Work out the finished part from the listing and answer in its coordinate system (mm). Face numbers are marked on the shaded views. A direction names the side the tool comes from. Give positions to 0.01 mm unless a question says otherwise; leave off trailing zeros. Loops run counter-clockwise (first coordinate to the right, second up) from the corner with the lowest first, then second, coordinate; pieces in that order, holes last. Notation, with made-up numbers: (84.5, -20.75) - (129.5, -20.75) arc R22 ccw to (129.5, 16.25) - close; hole circle Ø3 at (-26, 29). An arc over 180 degrees is marked (long way). One line per question, with ' | ' between items.
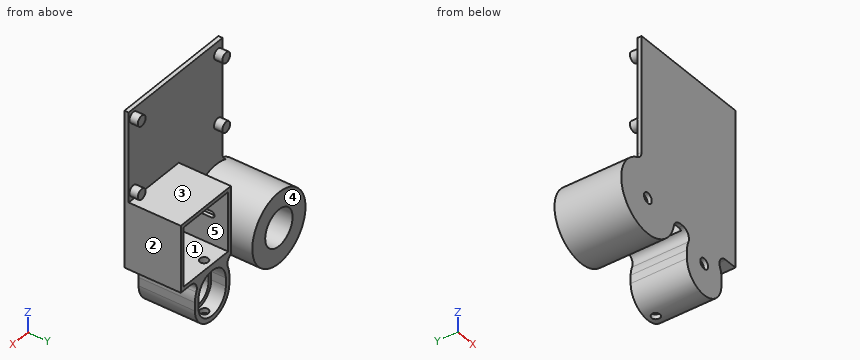
from build123d import *

# Parameters (mm, degrees)
SKETCH1_W                = 76.2
SKETCH1_H                = 95.25
BOSS_EXTRUDE1_DEPTH      = 2.54
SKETCH2_W                = 40.64
SKETCH2_H                = 40.64
BOSS_EXTRUDE2_DEPTH      = 31.75
SKETCH3_W                = 36.068
SKETCH3_H                = 36.068
CUT_EXTRUDE1_DEPTH       = 31.75
SKETCH4_R                = 3.175
BOSS_EXTRUDE3_DEPTH      = 5.08
CUT_EXTRUDE2_REACH       = 42.64
BOSS_EXTRUDE4_DEPTH      = 31.75
BOSS_EXTRUDE4_DEPTH_BACK = 2.54
FILLET1_R                = 5.08
CUT_EXTRUDE3_DEPTH       = 31.75
CUT_EXTRUDE4_DEPTH       = 8.89
SKETCH9_R                = 21.59
BOSS_EXTRUDE5_DEPTH      = 38.1
BOSS_EXTRUDE5_DEPTH_BACK = 2.54
SKETCH10_R               = 11.1125
CUT_EXTRUDE5_DEPTH       = 38.1
CUT_EXTRUDE6_REACH       = 4.54
SKETCH11_R               = 3.175
FILLET2_R                = 5.08
SKETCH13_R               = 2.5527
CUT_EXTRUDE7_DEPTH       = 35.036


with BuildPart() as part:
    # Sketch1 → Boss-Extrude1 (new body)
    with BuildSketch(Plane(origin=(0, 0, 0), x_dir=(1, 0, 0), z_dir=(0, 1, 0))):
        Rectangle(SKETCH1_W, SKETCH1_H)
    extrude(amount=BOSS_EXTRUDE1_DEPTH)

    # Sketch2 → Boss-Extrude2 (add)
    with BuildSketch(Plane(origin=(0, 2.54, 0), x_dir=(1, 0, 0), z_dir=(0, 1, 0))):
        with Locations((17.78, 27.305)):
            Rectangle(SKETCH2_W, SKETCH2_H)
    extrude(amount=BOSS_EXTRUDE2_DEPTH)

    # Sketch3 → Cut-Extrude1 (cut)
    with BuildSketch(Plane(origin=(0, 34.29, 0), x_dir=(1, 0, 0), z_dir=(0, 1, 0))):
        with Locations((17.78, 27.305)):
            Rectangle(SKETCH3_W, SKETCH3_H)
    extrude(amount=-CUT_EXTRUDE1_DEPTH, mode=Mode.SUBTRACT)

    # Sketch4 → Boss-Extrude3 (add)
    with BuildSketch(Plane(origin=(0, 2.54, 0), x_dir=(1, 0, 0), z_dir=(0, 1, 0))):
        with Locations(Location((34.29, 1.905, 0), (0, 0, 90))):  # turned: the seam where the file's is
            Circle(SKETCH4_R)
        with Locations(Location((34.29, -42.545, 0), (0, 0, 90))):  # turned: the seam where the file's is
            Circle(SKETCH4_R)
        with Locations(Location((-34.29, 1.905, 0), (0, 0, 90))):  # turned: the seam where the file's is
            Circle(SKETCH4_R)
        with Locations(Location((-34.29, -40.148547917, 0), (0, 0, 90))):  # turned: the seam where the file's is
            Circle(SKETCH4_R)
    extrude(amount=BOSS_EXTRUDE3_DEPTH)

    # Sketch5 → Cut-Extrude2 (cut, up to next)
    with BuildSketch(Plane.ZY.offset(2.54), mode=Mode.PRIVATE) as cut_extrude2_sk1:
        with BuildLine():
            Line((-29.21, 24.13), (-29.21, 5.08))
            ThreePointArc((-29.21, 5.08), (-27.305, 3.175), (-25.4, 5.08))
            Line((-25.4, 5.08), (-25.4, 24.13))
            ThreePointArc((-25.4, 24.13), (-27.305, 26.035), (-29.21, 24.13))
        make_face()
    cut_extrude2_tool1 = extrude(cut_extrude2_sk1.sketch, amount=-CUT_EXTRUDE2_REACH, mode=Mode.PRIVATE) & part.part
    add(cut_extrude2_tool1.solids().sort_by_distance((-2.54, 14.605, -27.305))[0], mode=Mode.SUBTRACT)

    # Sketch6 → Boss-Extrude4 (add, two sides)
    with BuildSketch(Plane(origin=(0, 2.54, 0), x_dir=(1, 0, 0), z_dir=(0, 1, 0))) as boss_extrude4_sk:
        with BuildLine():
            Line((26.67, 60.325), (26.67, 65.405))
            ThreePointArc((26.67, 65.405), (12.7, 79.375), (-1.27, 65.405))
            Line((-1.27, 65.405), (-1.27, 60.325))
            ThreePointArc((-1.27, 60.325), (12.7, 46.355), (26.67, 60.325))
        make_face()
    extrude(amount=BOSS_EXTRUDE4_DEPTH)
    extrude(boss_extrude4_sk.sketch, amount=-BOSS_EXTRUDE4_DEPTH_BACK)

    # Fillet1
    fillet1_edges = [part.edges().sort_by_distance(p)[0] for p in [
        (18.519871133, 17.145, -47.625),
        (6.880128867, 17.145, -47.625),
    ]]
    fillet(fillet1_edges, radius=FILLET1_R)

    # Sketch7 → Cut-Extrude3 (cut)
    with BuildSketch(Plane(origin=(0, 34.29, 0), x_dir=(1, 0, 0), z_dir=(0, 1, 0))):
        with BuildLine():
            Line((21.59, 60.325), (21.59, 65.405))
            ThreePointArc((21.59, 65.405), (12.7, 74.295), (3.81, 65.405))
            Line((3.81, 65.405), (3.81, 60.325))
            ThreePointArc((3.81, 60.325), (12.7, 51.435), (21.59, 60.325))
        make_face()
    extrude(amount=-CUT_EXTRUDE3_DEPTH, mode=Mode.SUBTRACT)

    # Sketch8 → Cut-Extrude4 (cut)
    with BuildSketch(Plane(origin=(0, 34.29, 0), x_dir=(1, 0, 0), z_dir=(0, 1, 0))):
        with BuildLine():
            Line((23.8125, 60.325), (23.8125, 65.405))
            ThreePointArc((23.8125, 65.405), (12.7, 76.5175), (1.5875, 65.405))
            Line((1.5875, 65.405), (1.5875, 60.325))
            ThreePointArc((1.5875, 60.325), (12.7, 49.2125), (23.8125, 60.325))
        make_face()
    extrude(amount=-CUT_EXTRUDE4_DEPTH, mode=Mode.SUBTRACT)

    # Sketch9 → Boss-Extrude5 (add, two sides)
    with BuildSketch(Plane(origin=(0, 2.54, 0), x_dir=(1, 0, 0), z_dir=(0, 1, 0))) as boss_extrude5_sk:
        with Locations(Location((-33.02, 47.625, 0), (0, 0, 270))):  # turned: the seam where the file's is
            Circle(SKETCH9_R)
    extrude(amount=BOSS_EXTRUDE5_DEPTH)
    extrude(boss_extrude5_sk.sketch, amount=-BOSS_EXTRUDE5_DEPTH_BACK)

    # Sketch10 → Cut-Extrude5 (cut)
    with BuildSketch(Plane(origin=(0, 40.64, 0), x_dir=(1, 0, 0), z_dir=(0, 1, 0))):
        with Locations(Location((-33.02, 47.625, 0), (0, 0, 270))):  # turned: the seam where the file's is
            Circle(SKETCH10_R)
    extrude(amount=-CUT_EXTRUDE5_DEPTH, mode=Mode.SUBTRACT)

    # Sketch11 → Cut-Extrude6 (cut, up to next)
    with BuildSketch(Plane(origin=(0, 2.54, 0), x_dir=(1, 0, 0), z_dir=(0, 1, 0)), mode=Mode.PRIVATE) as cut_extrude6_sk1:
        with Locations(Location((12.7, 60.325, 0), (0, 0, 270))):  # turned: the seam where the file's is
            Circle(SKETCH11_R)
    cut_extrude6_tool1 = extrude(cut_extrude6_sk1.sketch, amount=-CUT_EXTRUDE6_REACH, mode=Mode.PRIVATE) & part.part
    add(cut_extrude6_tool1.solids().sort_by_distance((12.7, 2.54, -60.325))[0], mode=Mode.SUBTRACT)
    # Sketch11 → Cut-Extrude6 (cut, up to next)
    with BuildSketch(Plane(origin=(0, 2.54, 0), x_dir=(1, 0, 0), z_dir=(0, 1, 0)), mode=Mode.PRIVATE) as cut_extrude6_sk2:
        with Locations(Location((-33.02, 47.625, 0), (0, 0, 270))):  # turned: the seam where the file's is
            Circle(SKETCH11_R)
    cut_extrude6_tool2 = extrude(cut_extrude6_sk2.sketch, amount=-CUT_EXTRUDE6_REACH, mode=Mode.PRIVATE) & part.part
    add(cut_extrude6_tool2.solids().sort_by_distance((-33.02, 2.54, -47.625))[0], mode=Mode.SUBTRACT)

    # Fillet2
    fillet2_edges = [part.edges().sort_by_distance(p)[0] for p in [
        (-11.43, 1.27, -47.625),
        (-38.1, 1.27, -26.641156215),
    ]]
    fillet(fillet2_edges, radius=FILLET2_R)

    # Sketch13 → Cut-Extrude7 (cut, through all)
    with BuildSketch(Plane.XY.offset(-45.339)):
        with Locations((12.446, 29.21)):
            Circle(SKETCH13_R)
    extrude(amount=-CUT_EXTRUDE7_DEPTH, mode=Mode.SUBTRACT)


solid = part.part
1. Which of the six approach directions +Z, -Z, +X, -X, +Y, -Y give full straight-line access (tool end or side, diameter ignored) to the marked faces 4 and 5?
Evaluation:
face 4: +Z, -Z, +X, -X, +Y | face 5: +Y
2. Find section C-C on x = 34.29. Write down the section's boundary in (y, z) (3 decimals), then the cut area to 3 significant figures.
Evaluation:
outline: (0, -47.625) - (34.29, -47.625) - (34.29, -45.339) - (2.54, -45.339) - (2.54, -9.271) - (34.29, -9.271) - (34.29, -6.985) - (2.54, -6.985) - (2.54, -5.08) - (7.62, -5.08) - (7.62, 1.27) - (2.54, 1.27) - (2.54, 39.37) - (7.62, 39.37) - (7.62, 45.72) - (2.54, 45.72) - (2.54, 47.625) - (0, 47.625) - close | area: 452 mm2
3. Determine the mould class of the marked faces 1, 2 and 3 for opening direction X: +X half, -X half, draft (parallel to the pull), parting line (faces both ways), or undercut.
Evaluation:
face 1: undercut | face 2: +X half | face 3: draft
4. Flat-ended cylindrical pins translate along their axes: pin 1 (6 mm diameter, centred on x = 26, z = -52, fed in from +Y); pin 2 (0.7 mm diameter, centred on x = -1, y = 16.5, fed in from +Z) (3 decimals); pin 3 (5 mm diameter, centred on x = -5, y = 27, fed in from -Z); pin 4 (4 mm diameter, centred on x = -33.02, z = -47.625, fed in from +Y). Find the tip coordinate at first contact, or state that the pin passes through.
Evaluation:
pin 1: y = 34.29 | pin 2: z = -6.985 | pin 3: z = -48.16 | pin 4: through
5. Consider L1, parallel to X at y = 13, z = -34.5; L2, parallel to Z at x = 15.5, y = 30.5 (3 decimals); L3, parallel to X at y = 18, z = -44. Determine where each line is inside the solid, lowest interval first.
Evaluation:
L1: -50.16 to -15.88, -2.54 to -0.25, 35.81 to 38.1 | L2: -79.092 to -76.159, -49.571 to -45.339, -9.271 to -6.985 | L3: -54.3 to -43.52, -22.52 to -11.74, -2.54 to -0.25, 35.81 to 38.1
6. Find section A-A on y = 16. Write down the section's boundary in (x, z) (1 decimal).
Evaluation:
outline: circle Ø43.2 at (-33, -47.6); (-2.5, -48.1) arc R5.1 cw to (-0.1, -54.7) arc R14 ccw to (-1.3, -60.3) - (-1.3, -65.4) arc R14 ccw to (26.7, -65.4) - (26.7, -60.3) arc R14 ccw to (25.5, -54.7) arc R5.1 cw to (30.2, -47.6) - (38.1, -47.6) - (38.1, -7) - (-2.5, -7) - (-2.5, -25.4) - (-0.3, -25.4) - (-0.3, -9.3) - (35.8, -9.3) - (35.8, -45.3) - (-0.3, -45.3) - (-0.3, -29.2) - (-2.5, -29.2) - close; hole circle Ø22.2 at (-33, -47.6); hole (3.8, -65.4) arc R8.9 ccw to (21.6, -65.4) - (21.6, -60.3) arc R8.9 ccw to (3.8, -60.3) - close
7. Find section D-D on y = 29.21. State how many separate pieces and enclosed holes the cut face has, then the cut area to 3 significant figures.
Evaluation:
separate pieces: 2 | enclosed holes: 1 | area: 1,680 mm2
8. Find section B-B on z = -67. Write down the section's boundary in (x, y), then the cut area to 3 significant figures.
Evaluation:
outline: (-42.55, 0) - (-23.49, 0) - (-23.49, 40.64) - (-42.55, 40.64) - close; (-1.18, 0) - (26.58, 0) - (26.58, 34.29) - (23.7, 34.29) - (23.7, 25.4) - (21.45, 25.4) - (21.45, 2.54) - (3.95, 2.54) - (3.95, 25.4) - (1.7, 25.4) - (1.7, 34.29) - (-1.18, 34.29) - close | area: 1,130 mm2
